```python
from build123d import *

# Parameters (mm, degrees)
PAD010_DEPTH    = 12.5
SKETCH018_R     = 1.4
POCKET006_DEPTH = 15.001
POCKET007_DEPTH = 2
POCKET008_DEPTH = 2.5
POCKET009_DEPTH = 15.001
SKETCH023_R     = 1.15
POCKET010_DEPTH = 12.001
POCKET011_DEPTH = 10.801
POCKET012_DEPTH = 12.001


with BuildPart() as part:
    # Sketch016 → Pad010 (new body, symmetric)
    with BuildSketch(Plane.YZ):
        Polygon((0, 0), (0, 15), (2.6, 15), (2.6, 8.6), (12, 6.1), (12, 0), align=None)
    extrude(amount=PAD010_DEPTH, both=True)

    # Sketch018 → Pocket006 (cut, through all)
    with BuildSketch(Plane.XY):
        with Locations((-4, 7)):
            Circle(SKETCH018_R)
        with Locations((4, 7)):
            Circle(SKETCH018_R)
    extrude(amount=POCKET006_DEPTH, mode=Mode.SUBTRACT)

    # Sketch019 (on DatumPlane) → Pocket007 (cut)
    with BuildSketch(Plane.XY.offset(1.6)):
        Polygon((-4, 10.002221), (-6.6, 8.501111), (-6.6, 5.498889), (-4, 3.997779), (-1.4, 5.498889), (-1.4, 8.501111), align=None)
        Polygon((4, 10.002221), (1.4, 8.501111), (1.4, 5.498889), (4, 3.997779), (6.6, 5.498889), (6.6, 8.501111), align=None)
    extrude(amount=POCKET007_DEPTH, mode=Mode.SUBTRACT)

    # Sketch020 (on DatumPlane) → Pocket008 (cut)
    with BuildSketch(Plane.XY.offset(3.6)):
        Polygon((-4, 3.997779), (-1.4, 5.498889), (-1.4, 8.501111), (-1.4, 20.501111), (-6.6, 20.501111), (-6.6, 8.501111), (-6.6, 5.498889), align=None)
        Polygon((4, 3.997779), (6.6, 5.498889), (6.6, 8.501111), (6.6, 20.501111), (1.4, 20.501111), (1.4, 8.501111), (1.4, 5.498889), align=None)
    extrude(amount=POCKET008_DEPTH, mode=Mode.SUBTRACT)

    # Sketch021 → Pocket009 (cut, through all)
    with BuildSketch(Plane.XY):
        with BuildLine():
            Line((-12.5, 0), (-12.5, 1.6))
            ThreePointArc((-11.5, 2.6), (-12.207107, 2.307107), (-12.5, 1.6))
            Line((-11.5, 2.6), (-9.6, 2.6))
            ThreePointArc((-9.6, 2.6), (-8.892893, 2.892893), (-8.6, 3.6))
            Line((-8.6, 3.6), (-8.6, 11))
            ThreePointArc((-7.6, 12), (-8.307107, 11.707107), (-8.6, 11))
            Line((-7.6, 12), (7.6, 12))
            ThreePointArc((8.6, 11), (8.307107, 11.707107), (7.6, 12))
            Line((8.6, 11), (8.6, 3.6))
            ThreePointArc((8.6, 3.6), (8.892893, 2.892893), (9.6, 2.6))
            Line((9.6, 2.6), (11.5, 2.6))
            ThreePointArc((12.5, 1.6), (12.207107, 2.307107), (11.5, 2.6))
            Line((12.5, 1.6), (12.5, 0))
            Line((12.5, 0), (22.5, 0))
            Line((22.5, 0), (22.5, 22))
            Line((22.5, 22), (-22.5, 22))
            Line((-22.5, 22), (-22.5, 0))
            Line((-12.5, 0), (-22.5, 0))
        make_face()
    extrude(amount=POCKET009_DEPTH, mode=Mode.SUBTRACT)

    # Sketch023 → Pocket010 (cut, through all)
    with BuildSketch(Plane.XZ):
        with Locations((-10, 11)):
            Circle(SKETCH023_R)
        with Locations((10, 11)):
            Circle(SKETCH023_R)
    extrude(amount=-POCKET010_DEPTH, mode=Mode.SUBTRACT)

    # Sketch024 (on DatumPlane) → Pocket011 (cut, through all)
    with BuildSketch(Plane.XZ.offset(-1.2)):
        Polygon((7.575129, 11), (8.787564, 8.9), (11.212436, 8.9), (21.212436, 8.9), (21.212436, 13.1), (11.212436, 13.1), (8.787564, 13.1), align=None)
        Polygon((-7.575129, 11), (-8.787564, 13.1), (-11.212436, 13.1), (-21.212436, 13.1), (-21.212436, 8.9), (-11.212436, 8.9), (-8.787564, 8.9), align=None)
    extrude(amount=-POCKET011_DEPTH, mode=Mode.SUBTRACT)

    # Sketch025 → Pocket012 (cut, through all)
    with BuildSketch(Plane.XZ):
        with BuildLine():
            Line((-12.5, 0), (-12.5, 13))
            ThreePointArc((-10.5, 15), (-11.914214, 14.414214), (-12.5, 13))
            Line((-6.75, 15), (-10.5, 15))
            ThreePointArc((-6.25, 14.5), (-6.396447, 14.853553), (-6.75, 15))
            Line((-6.25, 13.5), (-6.25, 14.5))
            ThreePointArc((-6.25, 13.5), (-6.103553, 13.146447), (-5.75, 13))
            Line((-5.75, 13), (5.75, 13))
            ThreePointArc((5.75, 13), (6.103553, 13.146447), (6.25, 13.5))
            Line((6.25, 13.5), (6.25, 14.5))
            ThreePointArc((6.75, 15), (6.396447, 14.853553), (6.25, 14.5))
            Line((6.75, 15), (10.5, 15))
            ThreePointArc((12.5, 13), (11.914214, 14.414214), (10.5, 15))
            Line((12.5, 13), (12.5, 0))
            Line((12.5, 0), (17.5, 0))
            Line((17.5, 0), (17.5, 20))
            Line((17.5, 20), (-17.5, 20))
            Line((-17.5, 20), (-17.5, 0))
            Line((-17.5, 0), (-12.5, 0))
        make_face()
    extrude(amount=-POCKET012_DEPTH, mode=Mode.SUBTRACT)


solid = part.part
```
Can you work these out from the model? Positions are in its coordinate system, mm. A direction names the side the tool comes from. Coordinates: 2 decimals unless noted, no trailing zeros. Order: outer loops, then holes, each group sorted by start corner. A loop starts at its lowest first (then second) coordinate and runs counter-clockwise, first axis right, second up.
1. Thinking about a two-plate mould opening in Y: for faces 6 (the face through (-2.68, 9.24, 2.59)), 7 (the face through (8.885, 2.901, 4.24)), 8 (the face through (-8.6, 7, 4)), which applies, +Y half, -Y half, draft (parallel to the pull), parting line (faces both ways), or undercut?
2. I need wall thicknesses on line 1 (X direction, y = 8.75, z = 4); line 2 (Y direction, x = -4, z = 0.3); line 3 (X direction, y = 7, z = 0.55). Which ranges of each line are inside material? Lowest first, please.
3. For faces 1 (the face through (11, 2, 8.9)), 2 (the face through (0, 1, 13)), 3 (the face through (2.718, 9.262, 2.586)), 4 (the face through (0, 12, 2)), 5 (the face through (-8.19, 1.89, 9.935)), which set-ups out of +Z, -Z, +X, -X, +Y, -Y let a thin tool reach every point of the face, with its end or its side?
4. If we section it at D-D (z = 2.75): Please give me the cut outline in (x, y).
5. If we section it at C-C (y = 7.75): Please give me the cut outline in (x, z).
6. I'm going to push flat-ended pins straight in: pin 1 (5.5 mm diameter, centred on x = 3, y = 5.5, fed in from +Z); pin 2 (4.5 mm diameter, centred on x = 10.5, z = 10.5, fed in from +Y); pin 3 (2 mm diameter, centred on y = 7.5, z = 3.5, fed in from -X). Where does each tip first touch, or does it pass through?
7. If we section it at B-B (z = 4.5): Please give me the cut outline in (x, y).
8. If we section it at A-A (x = 10): Please give me the cut outline in (y, z).
Entries:
1. face 6: undercut
1. face 7: +Y half
1. face 8: draft
2. line 1: x = -8.6 to -6.6, -1.4 to 1.4, 6.6 to 8.6
2. line 2: y = 0 to 5.6, 8.4 to 12
2. line 3: x = -8.6 to -5.4, -2.6 to 2.6, 5.4 to 8.6
3. face 1: +X, +Y
3. face 2: +Z, +Y, -Y
3. face 3: none
3. face 4: +Z, -Z, +X, -X, +Y
3. face 5: -X, +Y
4. outline: (-12.5, 0) - (12.5, 0) - (12.5, 1.6) arc R1 ccw to (11.5, 2.6) - (9.6, 2.6) arc R1 cw to (8.6, 3.6) - (8.6, 11) arc R1 ccw to (7.6, 12) - (-7.6, 12) arc R1 ccw to (-8.6, 11) - (-8.6, 3.6) arc R1 cw to (-9.6, 2.6) - (-11.5, 2.6) arc R1 ccw to (-12.5, 1.6) - close; hole (-6.6, 5.5) - (-4, 4) - (-1.4, 5.5) - (-1.4, 8.5) - (-4, 10) - (-6.6, 8.5) - close; hole (1.4, 5.5) - (4, 4) - (6.6, 5.5) - (6.6, 8.5) - (4, 10) - (1.4, 8.5) - close
5. outline: (-8.6, 0) - (-5.18, 0) - (-5.18, 1.6) - (-6.6, 1.6) - (-6.6, 6.1) - (-5.18, 6.1) - (-5.18, 7.23) - (-8.6, 7.23) - close; (-2.82, 0) - (2.82, 0) - (2.82, 1.6) - (1.4, 1.6) - (1.4, 6.1) - (2.82, 6.1) - (2.82, 7.23) - (-2.82, 7.23) - (-2.82, 6.1) - (-1.4, 6.1) - (-1.4, 1.6) - (-2.82, 1.6) - close; (5.18, 0) - (8.6, 0) - (8.6, 7.23) - (5.18, 7.23) - (5.18, 6.1) - (6.6, 6.1) - (6.6, 1.6) - (5.18, 1.6) - close
6. pin 1: stops at z = 8.56
6. pin 2: stops at y = 2.64
6. pin 3: stops at x = -8.6
7. outline: (-12.5, 0) - (12.5, 0) - (12.5, 1.6) arc R1 ccw to (11.5, 2.6) - (9.6, 2.6) arc R1 cw to (8.6, 3.6) - (8.6, 11) arc R1 ccw to (7.6, 12) - (6.6, 12) - (6.6, 5.5) - (4, 4) - (1.4, 5.5) - (1.4, 12) - (-1.4, 12) - (-1.4, 5.5) - (-4, 4) - (-6.6, 5.5) - (-6.6, 12) - (-7.6, 12) arc R1 ccw to (-8.6, 11) - (-8.6, 3.6) arc R1 cw to (-9.6, 2.6) - (-11.5, 2.6) arc R1 ccw to (-12.5, 1.6) - close
8. outline: (0, 0) - (2.6, 0) - (2.6, 8.9) - (1.2, 8.9) - (1.2, 9.85) - (0, 9.85) - close; (0, 12.15) - (1.2, 12.15) - (1.2, 13.1) - (2.6, 13.1) - (2.6, 15) - (0, 15) - close
